Answer from the drawing. Dimensions are ordinates in mm from the lowest x, y and z of the part. A direction names the side the tool comes from. Give positions to 0.01 mm unless a question says otherwise; leave off trailing zeros. Order: outer loops, then holes, each group sorted by start corner. A loop starts at its lowest first (then second) coordinate and runs counter-clockwise, first axis right, second up. Notation, with made-up numbers: (-38, -26) -> (16, -26) arc R19 cw to (16, -12) -> close; hole circle Ø10 at (56, -37). An arc over 180 degrees is marked (long way). Answer as CSV lines item,"result". Start each with the question number.
1) Straight lines are drawn through the part: L1, parallel to Y at x = 3.5, z = 8.7 (1 decimal); L2, parallel to Y at x = 3.5, z = 0.3 (1 decimal); L3, parallel to Z at x = 1.75, y = 7 (1 decimal). For each, find the intervals that lie inside material, in ascending order. Write a range as from..to.
2) Find section A-A (z = 9). Determine the outline of the cut face in (x, y).
3) For the marked faces 1 and 2, determine the directions among +Z, -Z, +X, -X, +Y, -Y from which every point of the face is accessible in a straight line to the end or side of a thin tool.
4) Flat-ended cylindrical pins translate along their axes: pin 1 Ø1.9 at (x, y) = (1, 5) entering from -Z; pin 2 Ø1.1 at (x, y) = (2.5, 7.5) entering from -Z; pin 3 Ø1.9 at (x, y) = (6.5, 2.5) entering from -Z. Find the tip coordinate at first contact, or state that the pin passes through.
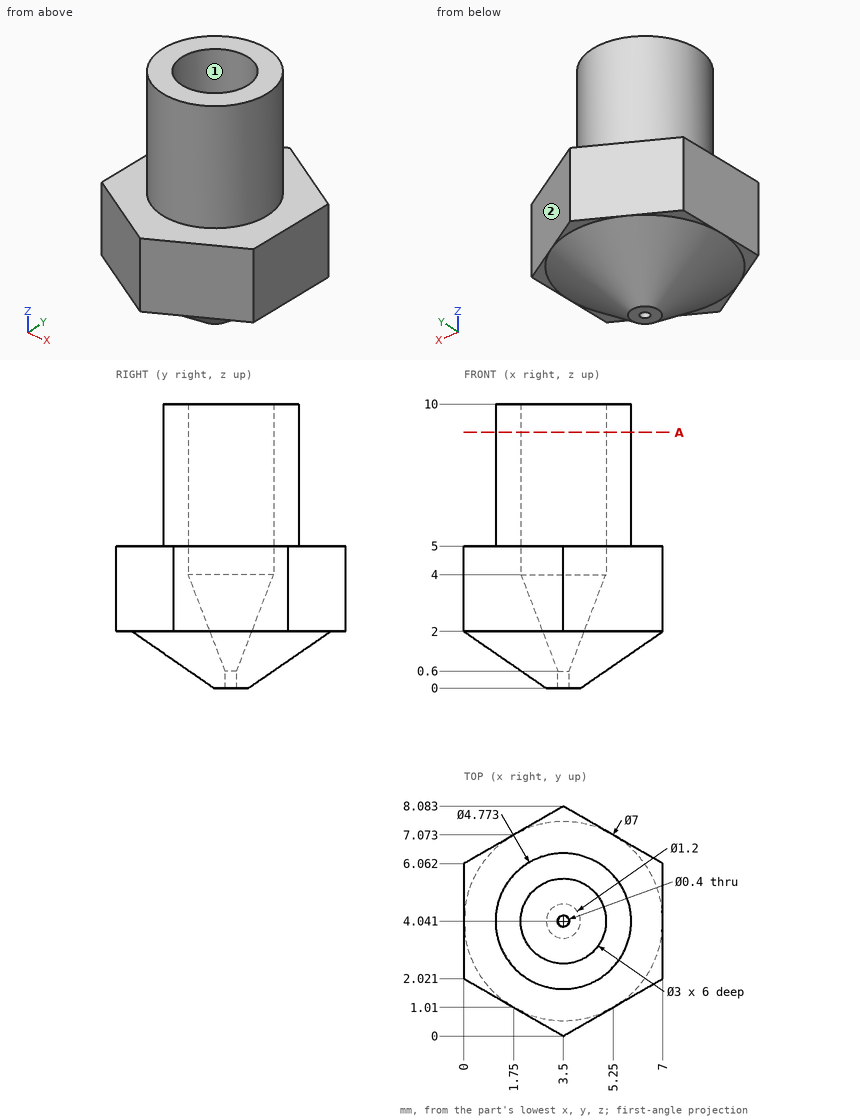
Findings below:
1,L1,"1.7..2.5, 5.5..6.4"
1,L2,"3..3.8, 4.2..5.1"
1,L3,"2..5"
2,outline,"circle Ø4.77 at (3.5, 4.04); hole circle Ø3 at (3.5, 4.04)"
3,face 1,"+Z"
3,face 2,"+Z, -Z, +X, +Y"
4,pin 1,"z = 0.78"
4,pin 2,"z = 1.69"
4,pin 3,"z = 1.26"
